Here's the drawing with two shaded views (mm, measured from the low corner). I have some questions. Round coordinates to 2 decimals unless told otherwise and drop trailing zeros. Loops run counter-clockwise (first coordinate to the right, second up) from the corner with the lowest first, then second, coordinate; pieces in that order, holes last. Notation, with made-up numbers: (78.25, 88.25) -> (131.25, 88.25) arc R23 cw to (131.25, 127.25) -> close; hole circle Ø8 at (88, 15). An arc over 180 degrees is marked (long way). Write each question's results on one line, items separated by ' | '.
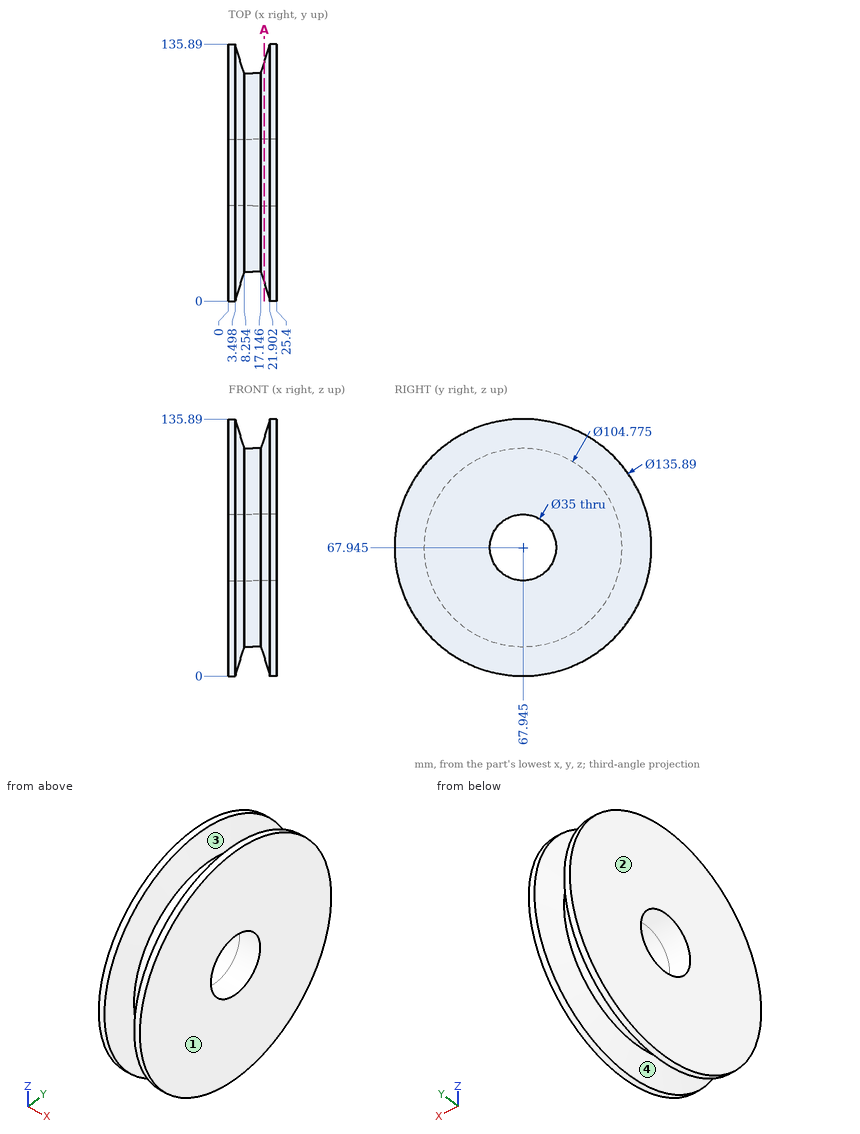
1. We'd pull the mould along X, two halves only. Please class the marked faces 1, 2, 3 and 4: pulls with the +X half, pulls with the -X half, needs draft (parallel to the pull), parting line crosses it, or undercut.
Final values:
face 1: pulls with the +X half | face 2: pulls with the -X half | face 3: undercut | face 4: undercut
2. Please list where these lines run through material, in increasing order: line 1 (Z direction, x = 10.25, y = 68.5); line 2 (X direction, y = 113, z = 38); line 3 (Z direction, x = 22.75, y = 74) (1 decimal). Write a range as from..to.
Final values:
line 1: 15.56..50.45, 85.44..120.33 | line 2: 0..7.73, 17.67..25.4 | line 3: 0.3..51.5, 84.4..135.6
3. Will these pins go through, and if not, where does the flat tip stop? pin 1 (12 mm diameter, centred on x = 16.5, y = 24.5, fed in from -Z); pin 2 (1.5 mm diameter, centred on x = 11.5, z = 90, fed in from +Y) (1 decimal).
Final values:
pin 1: z = 13.64 | pin 2: y = 115.8
4. If we section it at A-A (x = 19): List the corners of the cut face in (y, z) for me (1 decimal).
Final values:
outline: circle Ø116.9 at (67.9, 67.9); hole circle Ø35 at (67.9, 67.9)
